Part print with two shaded views. Sizes in mm from the minimum x, y, z corner. Round coordinates to 2 decimals unless told otherwise and drop trailing zeros. Loops run counter-clockwise (first coordinate to the right, second up) from the corner with the lowest first, then second, coordinate; pieces in that order, holes last.
(1) Cut at D-D on z = 75. List the corners of the cut face in (x, y), then the cut area to 3 significant figures.
(2) Cut at B-B on x = 3.35. List the corners of the cut face in (y, z) (3 decimals), then the cut area to 3 significant figures.
(3) Flat gauge pin, fed straight in: pin 1 (2 mm diameter, centred on x = 3, y = 7, fed in from +Z). Where does the tip first touch, or does it go through?
(4) Cut at A-A on y = 15. List the corners of the cut face in (x, z) (3 decimals), then the cut area to 3 significant figures.
(5) Probe probe 1 along Y at (x, z) = (3, 75); probe 2 along Y at (x, z) = (2.75, 49); probe 3 along Z at (x, y) = (0.45, 7). List the from-to ranges inside material, lowest first.
(6) Cut at C-C on z = 40.25. List the corners of the cut face in (x, y) (3 decimals).
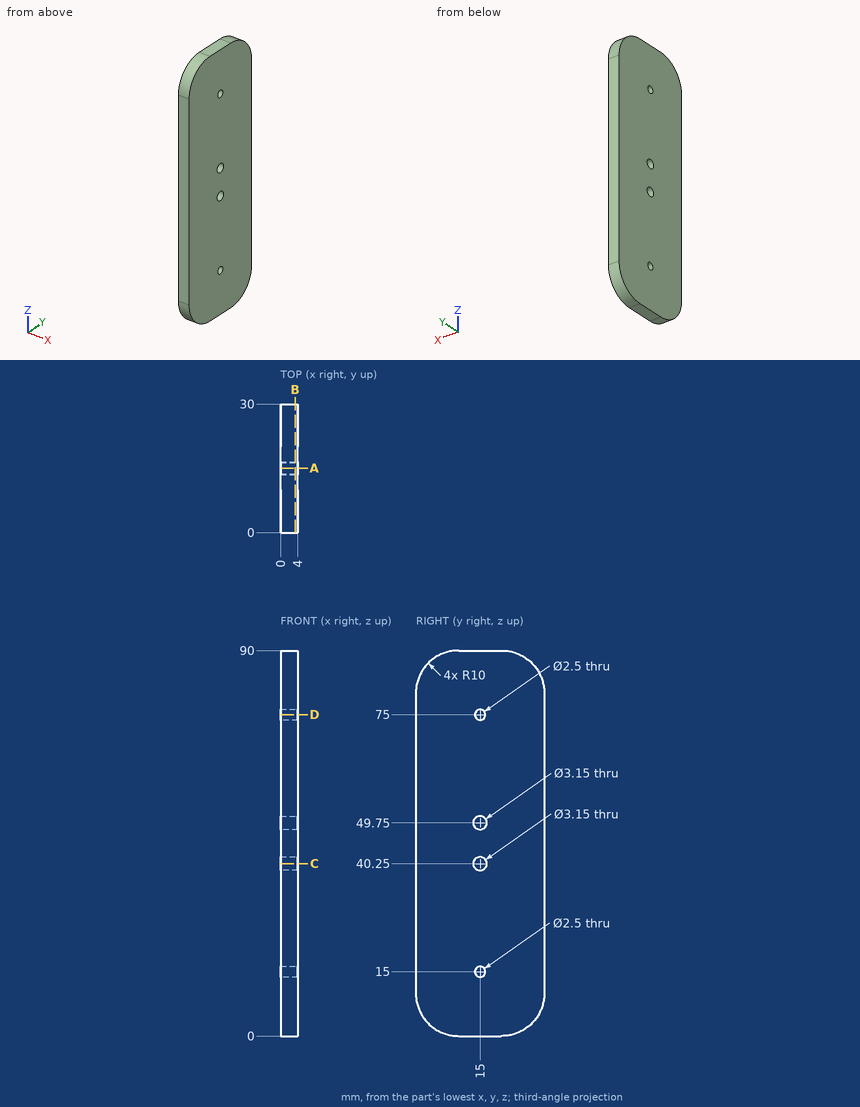
Final values:
1. outline: (0, 0) - (4, 0) - (4, 13.75) - (0, 13.75) - close; (0, 16.25) - (4, 16.25) - (4, 30) - (0, 30) - close
1. area: 110 mm2
2. outline: (0, 10) arc R10 ccw to (10, 0) - (20, 0) arc R10 ccw to (30, 10) - (30, 80) arc R10 ccw to (20, 90) - (10, 90) arc R10 ccw to (0, 80) - close; hole circle Ø3.15 at (15, 40.25); hole circle Ø3.15 at (15, 49.75); hole circle Ø2.5 at (15, 15); hole circle Ø2.5 at (15, 75)
2. area: 2,590 mm2
3. pin 1: stops at z = 89.8
4. outline: (0, 0) - (4, 0) - (4, 13.75) - (0, 13.75) - close; (0, 16.25) - (4, 16.25) - (4, 38.675) - (0, 38.675) - close; (0, 41.825) - (4, 41.825) - (4, 48.175) - (0, 48.175) - close; (0, 51.325) - (4, 51.325) - (4, 73.75) - (0, 73.75) - close; (0, 76.25) - (4, 76.25) - (4, 90) - (0, 90) - close
4. area: 315 mm2
5. probe 1: y = 0 to 13.75, 16.25 to 30
5. probe 2: y = 0 to 13.62, 16.38 to 30
5. probe 3: z = 0.46 to 89.54
6. outline: (0, 0) - (4, 0) - (4, 13.425) - (0, 13.425) - close; (0, 16.575) - (4, 16.575) - (4, 30) - (0, 30) - close
